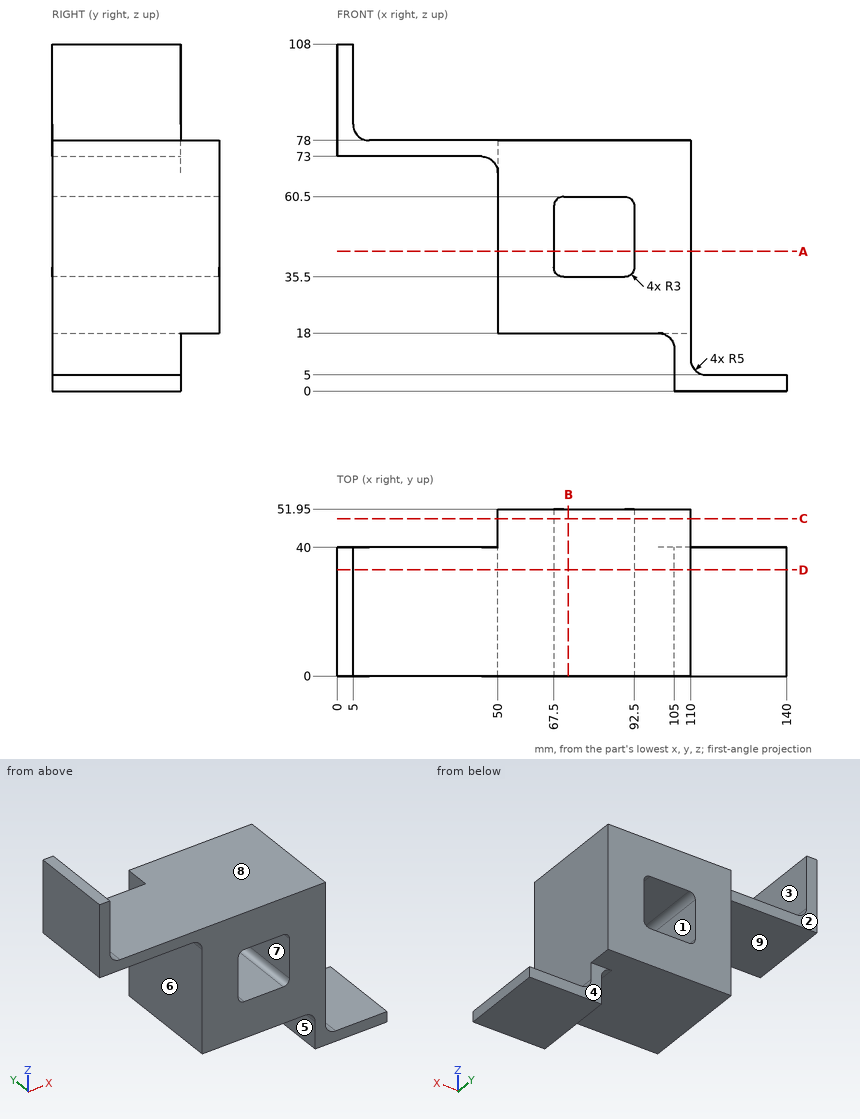
Here's the drawing with two shaded views (mm, measured from the low corner). I have some questions. A direction names the side the tool comes from. Round coordinates to 2 decimals unless told otherwise and drop trailing zeros. Loops run counter-clockwise (first coordinate to the right, second up) from the corner with the lowest first, then second, coordinate; pieces in that order, holes last. Notation, with made-up numbers: (62, 16) -> (96, 16) arc R32 cw to (96, 43) -> close; hole circle Ø2 at (82.5, -4). An arc over 180 degrees is marked (long way). Answer as CSV lines item,"result". Start each with the question number.
1. Imagine slicing it at A-A on z = 43.5. Write out the boundary of the cut face in (x, y).
2. For the marked faces 1, 2, 3, 4 and 5, which set-ups out of +Z, -Z, +X, -X, +Y, -Y let a thin tool reach every point of the face, with its end or its side?
3. If we mould it in two halves opening along Z, with no side actions, what happens to the marked faces 6, 7, 8 and 9? For each: pulls with the +Z half, pulls with the -Z half, needs draft (parallel to the pull), parting line crosses it, or undercut.
4. Imagine slicing it at B-B on x = 72. Write out the boundary of the cut face in (y, z).
5. I need wall thicknesses on probe 1 along X at (y, z) = (20.5, 53.5); probe 2 along Y at (x, z) = (39.5, 77); probe 3 along X at (y, z) = (25, 31.5). Which ranges of each line are inside material? Lowest first, please. Write a range as from..to.
6. I'm going to push flat-ended pins straight in: P1, Ø21, axis at y = 28, z = 45.5, coming from the -X side; P2, Ø4, axis at y = 8, z = 69.5, coming from the +X side; P3, Ø20, axis at x = 21.5, y = 15, coming from the -Z side. Where does each tip first touch, or does it pass through?
7. Imagine slicing it at D-D on y = 33. Write out the boundary of the cut face in (x, z), plus the area to 3 significant figures.
8. Imagine slicing it at C-C on y = 49. Write out the boundary of the cut face in (x, z).
Solution:
1,outline,"(50, 0) -> (67.5, 0) -> (67.5, 51.95) -> (50, 51.95) -> close; (92.5, 0) -> (110, 0) -> (110, 51.95) -> (92.5, 51.95) -> close"
2,face 1,"+Y, -Y"
2,face 2,"+Z, -Z, -X, +Y"
2,face 3,"+Z, +X, +Y, -Y"
2,face 4,"-Z, +X, -X, +Y"
2,face 5,"-Z, -X, +Y, -Y"
3,face 6,"needs draft"
3,face 7,"undercut"
3,face 8,"pulls with the +Z half"
3,face 9,"pulls with the -Z half"
4,outline,"(0, 18) -> (51.95, 18) -> (51.95, 35.5) -> (0, 35.5) -> close; (0, 60.5) -> (51.95, 60.5) -> (51.95, 78) -> (0, 78) -> close"
5,probe 1,"50..67.5, 92.5..110"
5,probe 2,"0..40"
5,probe 3,"50..110"
6,P1,"x = 50"
6,P2,"x = 110"
6,P3,"z = 73"
7,outline,"(0, 73) -> (45, 73) arc R5 cw to (50, 68) -> (50, 18) -> (100, 18) arc R5 cw to (105, 13) -> (105, 0) -> (140, 0) -> (140, 5) -> (115, 5) arc R5 cw to (110, 10) -> (110, 78) -> (10, 78) arc R5 cw to (5, 83) -> (5, 108) -> (0, 108) -> close; hole (67.5, 38.5) arc R3 ccw to (70.5, 35.5) -> (89.5, 35.5) arc R3 ccw to (92.5, 38.5) -> (92.5, 57.5) arc R3 ccw to (89.5, 60.5) -> (70.5, 60.5) arc R3 ccw to (67.5, 57.5) -> close"
7,area,"3,640 mm²"
8,outline,"(50, 18) -> (110, 18) -> (110, 78) -> (50, 78) -> close; hole (67.5, 38.5) arc R3 ccw to (70.5, 35.5) -> (89.5, 35.5) arc R3 ccw to (92.5, 38.5) -> (92.5, 57.5) arc R3 ccw to (89.5, 60.5) -> (70.5, 60.5) arc R3 ccw to (67.5, 57.5) -> close"
